Read the model definition and answer for the solid it produces. Units are mm, in the model's axes. Face numbers are marked on the shaded views. A direction names the side the tool comes from. Give positions to 0.01 mm unless a question says otherwise; leave off trailing zeros. Order: outer loops, then holes, each group sorted by start corner. A loop starts at its lowest first (then second) coordinate and runs counter-clockwise, first axis right, second up. Notation, with made-up numbers: (88.5, 70.25) -> (146.5, 70.25) arc R29 cw to (146.5, 90.25) -> close; hole circle Ø4 at (14, 45). An arc over 180 degrees is marked (long way). Answer as CSV lines item,"result". Start each with the question number.
1) Find section D-D (y = -12). Determine the outline of the cut face in (x, z), and give its area (3 significant figures).
2) Find section B-B (z = 5). Determine the outline of the cut face in (x, y), and give its area (3 significant figures).
3) Find section C-C (y = -87.5). Determine the outline of the cut face in (x, z), and give its area (3 significant figures).
4) Find section A-A (x = 7.5). Determine the outline of the cut face in (y, z).
5) Flat-ended cylindrical pins translate along their axes: pin 1 Ø3 at (x, z) = (-6, 19) entering from -Y; pin 2 Ø2 at (x, z) = (-85, 15.5) entering from +Y; pin 3 Ø1.5 at (x, z) = (-50.5, 11.5) entering from -Y; pin 4 Ø3 at (x, z) = (7.5, 5) entering from -Y. Find the tip coordinate at first contact, or state that the pin passes through.
6) Straight lines are drawn through the part: L1, parallel to Z at x = 7.5, y = -4.5; L2, parallel to Z at x = 7, y = -9; L3, parallel to X at y = -8.5, z = 25. For each, find the intervals that lie inside material, in ascending order. Write a range as from..to.
7) For the marked faces 4, 5 and 6, determine the directions among +Z, -Z, +X, -X, +Y, -Y from which every point of the face is accessible in a straight line to the end or side of a thin tool.
8) The mould has two halves that part along Y. Classify the marked faces 1, 2 and 3: +Y half, -Y half, draft (parallel to the pull), parting line (faces both ways), or undercut.
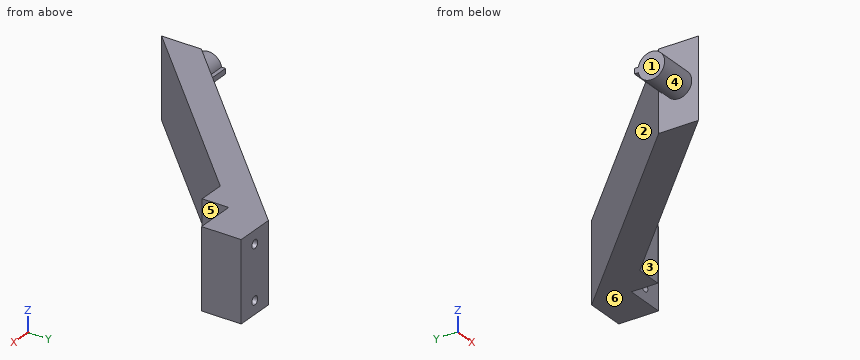
```python
from build123d import *

# Parameters (mm, degrees)
BOSS_EXTRUDE1_DEPTH     = 30
CUT_EXTRUDE1_DEPTH      = 128.769323392
CUT_EXTRUDE1_DEPTH_BACK = 15
SKETCH2_R               = 1.6
BOSS_EXTRUDE2_DEPTH     = 15


with BuildPart() as part:
    # Sketch1 → Boss-Extrude1 (new body)
    with BuildSketch(Plane.XY):
        Polygon((0, 0), (15, 0), (15, -15), (0, -15), (0, -25), (-10, -25), (-80, -95), (-80, -80), align=None)
    extrude(amount=BOSS_EXTRUDE1_DEPTH)

    # Sketch2 → Cut-Extrude1 (cut, two sides: drawn at the far end of the back side and taken through both)
    with BuildSketch(Plane(origin=(0, 0, 0), x_dir=(1, 0, 0), z_dir=(0, 1, 0)).offset(-CUT_EXTRUDE1_DEPTH_BACK)):
        with Locations(Location((7.5, -5, 0), (0, 0, 180))):
            Circle(SKETCH2_R)
        with Locations(Location((7.5, -25, 0), (0, 0, 180))):
            Circle(SKETCH2_R)
    extrude(amount=CUT_EXTRUDE1_DEPTH + CUT_EXTRUDE1_DEPTH_BACK, mode=Mode.SUBTRACT)

    # Sketch3 → Boss-Extrude2 (add)
    with BuildSketch(Plane.ZY.offset(80)):
        with BuildLine():
            Line((14, -82.601020514), (14, -81.101020514))
            Line((14, -81.101020514), (16, -81.101020514))
            Line((16, -81.101020514), (16, -82.601020514))
            ThreePointArc((16, -82.601020514), (15, -92.5), (14, -82.601020514))
        make_face()
    extrude(amount=BOSS_EXTRUDE2_DEPTH)


solid = part.part
```
Findings below:
1,outline,"(-12, 0) -> (15, 0) -> (15, 30) -> (-12, 30) -> close; hole circle Ø3.2 at (7.5, 5); hole circle Ø3.2 at (7.5, 25)"
1,area,"794 mm²"
2,outline,"(-80, -95) -> (-10, -25) -> (0, -25) -> (0, -15) -> (5.9, -15) -> (5.9, 0) -> (0, 0) -> (-80, -80) -> close; (9.1, -15) -> (15, -15) -> (15, 0) -> (9.1, 0) -> close"
2,area,"1,430 mm²"
3,outline,"(-95, 10) -> (-80, 10) -> (-80, 0) -> (-72.5, 0) -> (-72.5, 30) -> (-80, 30) -> (-80, 20) -> (-95, 20) -> close"
3,area,"375 mm²"
4,outline,"(-15, 0) -> (0, 0) -> (0, 3.4) -> (-15, 3.4) -> close; (-15, 6.6) -> (0, 6.6) -> (0, 23.4) -> (-15, 23.4) -> close; (-15, 26.6) -> (0, 26.6) -> (0, 30) -> (-15, 30) -> close"
5,pin 1,"y = -25"
5,pin 2,"y = -81.1"
5,pin 3,"y = -66.25"
5,pin 4,"through"
6,L1,"0..3.4, 6.6..23.4, 26.6..30"
6,L2,"0..3.48, 6.52..23.48, 26.52..30"
6,L3,"-8.5..5.9, 9.1..15"
7,face 4,"-X"
7,face 5,"+Z, -Z, +X, -Y"
7,face 6,"-Z, +X, -X, +Y, -Y"
8,face 1,"draft"
8,face 2,"+Y half"
8,face 3,"-Y half"
